Geometry: see drawing. Coordinates: mm, zero at the bounding-box minimum. Give positions to 0.01 mm unless a question says otherwise; leave off trailing zeros. Order: outer loops, then holes, each group sorted by start corner. A loop starts at its lowest first (then second) coordinate and runs counter-clockwise, first axis right, second up. Notation, with made-up numbers: (83, 48.5) - (113, 48.5) arc R32 ccw to (113, 85.5) - close; hole circle Ø1 at (57.25, 49). An arc over 180 degrees is marked (long way). Write each question's results on one line, items separated by ' | '. Start each with the question number.
Item 1: Mould query, pull axis X, two halves, no side actions, for the marked faces 1, 2 and 3. Classes: released by +X, released by -X, zero draft, split by the parting line, or undercut.
Item 2: Line query: line 1 along X through (y, z) = (1.5, 20) (1 decimal); line 2 along Z through (x, y) = (61.5, 4); line 3 along Y through (x, z) = (60, 34). Output: solid intervals per line, ascending.
Item 3: Section A-A on x = 86. Output: boundary loops of the cut face in (y, z), and give its area (3 significant figures).
Item 4: Section B-B on y = 3.25. Output: boundary loops of the cut face in (x, z) (1 decimal).
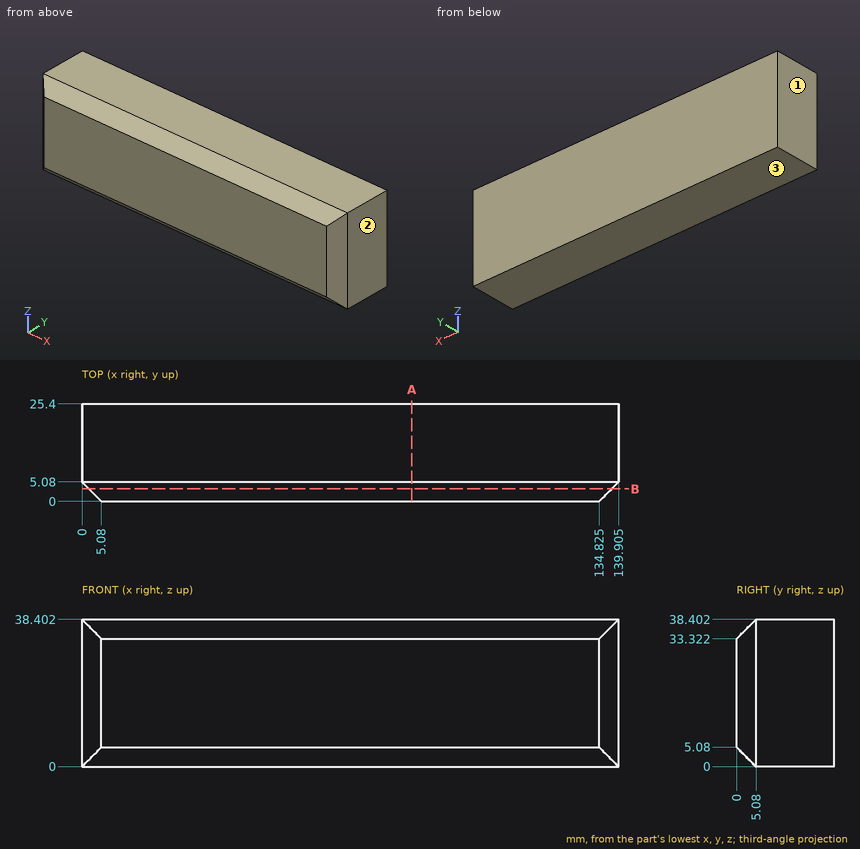
Evaluation:
1) face 1: released by -X | face 2: released by +X | face 3: zero draft
2) line 1: x = 3.6 to 136.3 | line 2: z = 1.08 to 37.32 | line 3: y = 0.68 to 25.4
3) outline: (0, 5.08) - (5.08, 0) - (25.4, 0) - (25.4, 38.4) - (5.08, 38.4) - (0, 33.32) - close | area: 950 mm^2
4) outline: (1.8, 1.8) - (138.1, 1.8) - (138.1, 36.6) - (1.8, 36.6) - close
